For this review, use the dimensioned drawing (mm, ordinates from the lowest corner) and the shaded views. A direction names the side the tool comes from. Give positions to 0.01 mm unless a question says otherwise; leave off trailing zeros. Loops run counter-clockwise (first coordinate to the right, second up) from the corner with the lowest first, then second, coordinate; pieces in that order, holes last. Notation, with made-up numbers: M 88,14 L 99,14 A29 ccw 99,46 Z; hole C 84.5,-19.5 d5. An arc over 180 degrees is marked long. Use CSV: the item, a comma, the result in double quotes. Start each with the question number.
1. Insertion check: P1, Ø2, axis at x = 112.5, z = 75, coming from the +Y side; P2, Ø17, axis at y = 53, z = 43, coming from the -X side; P3, Ø6, axis at x = 96, z = 44.5, coming from the -Y side. Each pin has a flat end and moves straight along its axis. Give the tip position at first contact, or say it passes through.
2. Take a section at A-A, the plane x = 76.2. Write out the cut boundary in (y, z), and give its area (3 significant figures).
3. The part is to be moulded in two halves that separate along X. For the marked faces 1, 2 and 3, say which applies: pulls with the +X half, pulls with the -X half, needs draft (parallel to the pull), parting line crosses it, or undercut.
4. Take a section at D-D, the plane x = 54. Write out the cut boundary in (y, z).
5. Tool access review of the marked faces 4, 5, 6 and 7: name each direction out of +Z, -Z, +X, -X, +Y, -Y from which nothing blocks a thin tool from reaching the whole face with its end or side.
6. Take a section at C-C, the plane z = 43. Write out the cut boundary in (x, y), and give its area (3 significant figures).
7. To check wall thickness, follow line 1 (Y direction, x = 76.2, z = 78); line 2 (X direction, y = 22.5, z = 41); line 3 (X direction, y = 38, z = 83). State the ranges of each line that lie inside material, in increasing order. Write a range as [from, to].
8. Take a section at B-B, the plane y = 65. Write out the cut boundary in (x, z).
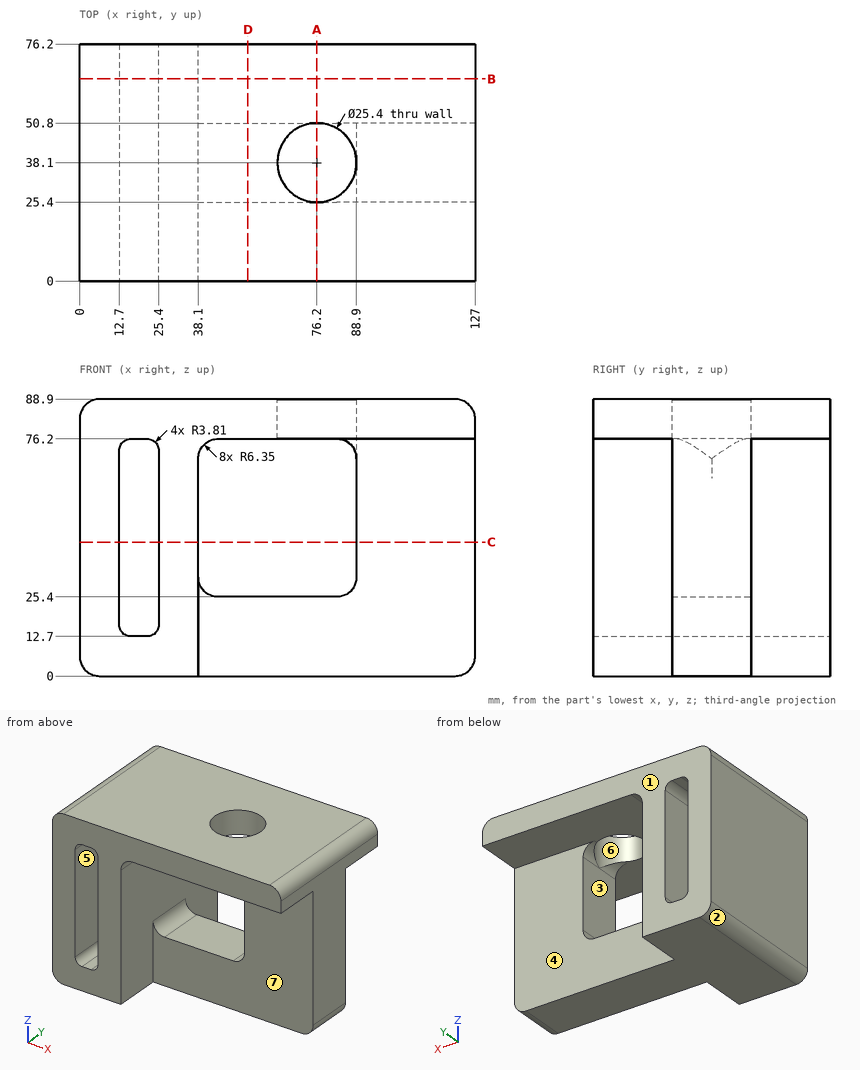
Result set:
1,P1,"y = 50.8"
1,P2,"x = 0"
1,P3,"y = 25.4"
2,outline,"M 0,76.2 L 25.4,76.2 L 25.4,88.9 L 0,88.9 Z; M 25.4,0 L 50.8,0 L 50.8,25.4 L 25.4,25.4 Z; M 50.8,76.2 L 76.2,76.2 L 76.2,88.9 L 50.8,88.9 Z"
2,area,"1,290 mm2"
3,face 1,"needs draft"
3,face 2,"pulls with the -X half"
3,face 3,"undercut"
4,outline,"M 0,76.2 L 76.2,76.2 L 76.2,88.9 L 0,88.9 Z; M 25.4,0 L 50.8,0 L 50.8,25.4 L 25.4,25.4 Z"
5,face 4,"-Z, +X, +Y"
5,face 5,"+Y, -Y"
5,face 6,"+Z"
5,face 7,"-Z, +X, -Y"
6,outline,"M 0,0 L 12.7,0 L 12.7,76.2 L 0,76.2 Z; M 25.4,0 L 38.1,0 L 38.1,76.2 L 25.4,76.2 Z; M 88.9,25.4 L 127,25.4 L 127,50.8 L 88.9,50.8 Z"
6,area,"2,900 mm2"
7,line 1,"[0, 25.4], [50.8, 76.2]"
7,line 2,"[0, 12.7], [25.4, 38.1]"
7,line 3,"[0.02, 63.5], [88.9, 126.98]"
8,outline,"M 0,6.35 A6.35 ccw 6.35,0 L 38.1,0 L 38.1,69.85 A6.35 cw 44.45,76.2 L 127,76.2 L 127,82.55 A6.35 ccw 120.65,88.9 L 6.35,88.9 A6.35 ccw 0,82.55 Z; hole M 12.7,16.51 A3.81 ccw 16.51,12.7 L 21.59,12.7 A3.81 ccw 25.4,16.51 L 25.4,72.39 A3.81 ccw 21.59,76.2 L 16.51,76.2 A3.81 ccw 12.7,72.39 Z"
